Could you check a few things on this model? Use its own coordinates, in mm. A direction names the side the tool comes from. Round coordinates to 2 decimals unless told otherwise and drop trailing zeros. Loops run counter-clockwise (first coordinate to the right, second up) from the corner with the lowest first, then second, coordinate; pieces in that order, holes last.
from build123d import *

# Parameters (mm, degrees)
F0_R     = 8.5
F1_DEPTH = 4
F2_R     = 5
F3_DEPTH = 100
F8_R     = 1.5
F9_DEPTH = 123.9


with BuildPart() as f1:
    # F0 (on Top) → F1 (new body)
    with BuildSketch(Plane.XY):
        Circle(F0_R)
    extrude(amount=F1_DEPTH)

    # F2 (on Top) → F3 (join)
    with BuildSketch(Plane.XY):
        Circle(F2_R)
    extrude(amount=F3_DEPTH)

    # F4 (on Right) → F5 (revolve)
    with BuildSketch(Plane.YZ):
        Polygon((3, 105), (0, 105), (0, 100), (4, 100), align=None)
    revolve(axis=Axis((0, 0, 102.5), (0, 0, -1)))

    # F6 (on Right) → F7 (revolve)
    with BuildSketch(Plane.YZ):
        with BuildLine():
            ThreePointArc((3, 105), (2.12132, 107.12132), (0, 108))
            Line((0, 108), (0, 105))
            Line((0, 105), (3, 105))
        make_face()
    revolve(axis=Axis((0, 0, 106.5), (0, 0, -1)))

    # F8 (on face) → F9 (cut)
    with BuildSketch(Plane(origin=(0, 0, 0), x_dir=(1, 0, 0), z_dir=(0, 0, -1))):
        Circle(F8_R)
    extrude(amount=-F9_DEPTH, mode=Mode.SUBTRACT)


solid = f1.part
Item 1: Will these pins go through, and if not, where does the flat tip stop? pin 1 (1.8 mm diameter, centred on x = 0, y = 0, fed in from +Z); pin 2 (10 mm diameter, centred on x = 6, z = 17.5, fed in from +Y); pin 3 (6 mm diameter, centred on x = -6, z = 42.5, fed in from -Y); pin 4 (3 mm diameter, centred on y = 0, z = 87.5, fed in from +X).
Results list:
pin 1: passes through
pin 2: stops at y = 4.9
pin 3: stops at y = -4
pin 4: stops at x = 5
Item 2: If we section it at C-C, the plane y = 7.25: Please give me the cut outline in (x, z).
Results list:
outline: (-4.44, 0) - (4.44, 0) - (4.44, 4) - (-4.44, 4) - close
Item 3: If I drill on line 1 along Y through (x, z) = (0, 28.5); line 2 along Z through (x, y) = (6.25, -1.25), over which ranges is the centre line in solid material (lowest first)?
Results list:
line 1: y = -5 to -1.5, 1.5 to 5
line 2: z = 0 to 4
Item 4: We'd pull the mould along X, two halves only. Please class faces 3 (the flat face through (2, 0, 0)), 4 (the cylindrical face through (-1.08, -4.88, 51.33)), 5 (the cylindrical face through (-1.5, -0.07, 53.05)): released by +X, released by -X, zero draft, split by the parting line, or undercut.
Results list:
face 3: zero draft
face 4: split by the parting line
face 5: undercut
Item 5: For faces 1 (the flat face through (4, -4, 4)), 2 (the cylindrical face through (4.57, 7.167, 1.972)), which set-ups out of +Z, -Z, +X, -X, +Y, -Y let a thin tool reach every point of the face, with its end or its side?
Results list:
face 1: +Z
face 2: +Z, -Z
Item 6: If we section it at A-A, the plane z = 81.5: Please give me the cut outline in (x, y).
Results list:
outline: circle Ø10 at (0, 0); hole circle Ø3 at (0, 0)
Item 7: If we section it at B-B, the plane x = 6.5: Please give me the cut outline in (y, z).
Results list:
outline: (-5.48, 0) - (5.48, 0) - (5.48, 4) - (-5.48, 4) - close
